from build123d import *

# Parameters (mm, degrees)
F0_R     = 1.905
F1_DEPTH = 12.7


with BuildPart() as f1:
    # F0 (on Top) → F1 (new body)
    with BuildSketch(Plane.XY):
        with BuildLine():
            ThreePointArc((114.3, 88.9), (106.860512, 106.860512), (88.9, 114.3))
            Line((88.9, 114.3), (3.175, 114.3))
            Line((3.175, 114.3), (3.175, 8.980256))
            ThreePointArc((3.175, 8.980256), (6.735192, 6.735192), (8.980256, 3.175))
            Line((8.980256, 3.175), (114.3, 3.175))
            Line((114.3, 3.175), (114.3, 88.9))
        make_face()
        with Locations((12.7, 12.7)):
            Circle(F0_R, mode=Mode.SUBTRACT)
        with Locations((38.1, 12.7)):
            Circle(F0_R, mode=Mode.SUBTRACT)
        with Locations((12.7, 38.1)):
            Circle(F0_R, mode=Mode.SUBTRACT)
        with Locations((38.1, 38.1)):
            Circle(F0_R, mode=Mode.SUBTRACT)
        with Locations((63.5, 12.7)):
            Circle(F0_R, mode=Mode.SUBTRACT)
        with Locations((88.9, 12.7)):
            Circle(F0_R, mode=Mode.SUBTRACT)
        with Locations((63.5, 38.1)):
            Circle(F0_R, mode=Mode.SUBTRACT)
        with Locations((88.9, 38.1)):
            Circle(F0_R, mode=Mode.SUBTRACT)
        with Locations((12.7, 63.5)):
            Circle(F0_R, mode=Mode.SUBTRACT)
        with Locations((38.1, 63.5)):
            Circle(F0_R, mode=Mode.SUBTRACT)
        with Locations((12.7, 88.9)):
            Circle(F0_R, mode=Mode.SUBTRACT)
        with Locations((38.1, 88.9)):
            Circle(F0_R, mode=Mode.SUBTRACT)
        with Locations((63.5, 63.5)):
            Circle(F0_R, mode=Mode.SUBTRACT)
        with Locations((88.9, 63.5)):
            Circle(F0_R, mode=Mode.SUBTRACT)
        with Locations((63.5, 88.9)):
            Circle(F0_R, mode=Mode.SUBTRACT)
        with Locations((88.9, 88.9)):
            Circle(F0_R, mode=Mode.SUBTRACT)
        with BuildLine():
            Line((3.175, 8.980256), (3.175, 114.3))
            Line((3.175, 114.3), (-3.175, 114.3))
            Line((-3.175, 114.3), (-3.175, 8.980256))
            ThreePointArc((-3.175, 8.980256), (0, 9.525), (3.175, 8.980256))
        make_face()
        with BuildLine():
            Line((-3.175, 8.980256), (-3.175, 114.3))
            Line((-3.175, 114.3), (-88.9, 114.3))
            ThreePointArc((-88.9, 114.3), (-106.860512, 106.860512), (-114.3, 88.9))
            Line((-114.3, 88.9), (-114.3, 3.175))
            Line((-114.3, 3.175), (-8.980256, 3.175))
            ThreePointArc((-8.980256, 3.175), (-6.735192, 6.735192), (-3.175, 8.980256))
        make_face()
        with Locations((-88.9, 12.7)):
            Circle(F0_R, mode=Mode.SUBTRACT)
        with Locations((-63.5, 12.7)):
            Circle(F0_R, mode=Mode.SUBTRACT)
        with Locations((-88.9, 38.1)):
            Circle(F0_R, mode=Mode.SUBTRACT)
        with Locations((-63.5, 38.1)):
            Circle(F0_R, mode=Mode.SUBTRACT)
        with Locations((-38.1, 12.7)):
            Circle(F0_R, mode=Mode.SUBTRACT)
        with Locations((-12.7, 12.7)):
            Circle(F0_R, mode=Mode.SUBTRACT)
        with Locations((-38.1, 38.1)):
            Circle(F0_R, mode=Mode.SUBTRACT)
        with Locations((-12.7, 38.1)):
            Circle(F0_R, mode=Mode.SUBTRACT)
        with Locations((-88.9, 63.5)):
            Circle(F0_R, mode=Mode.SUBTRACT)
        with Locations((-63.5, 63.5)):
            Circle(F0_R, mode=Mode.SUBTRACT)
        with Locations((-88.9, 88.9)):
            Circle(F0_R, mode=Mode.SUBTRACT)
        with Locations((-63.5, 88.9)):
            Circle(F0_R, mode=Mode.SUBTRACT)
        with Locations((-38.1, 63.5)):
            Circle(F0_R, mode=Mode.SUBTRACT)
        with Locations((-12.7, 63.5)):
            Circle(F0_R, mode=Mode.SUBTRACT)
        with Locations((-38.1, 88.9)):
            Circle(F0_R, mode=Mode.SUBTRACT)
        with Locations((-12.7, 88.9)):
            Circle(F0_R, mode=Mode.SUBTRACT)
        with BuildLine():
            Line((114.3, -3.175), (114.3, 3.175))
            Line((114.3, 3.175), (8.980256, 3.175))
            ThreePointArc((8.980256, 3.175), (9.387826, 1.610696), (9.525, 0))
            ThreePointArc((9.525, 0), (9.387826, -1.610696), (8.980256, -3.175))
            Line((8.980256, -3.175), (114.3, -3.175))
        make_face()
        with BuildLine():
            Line((114.3, -88.9), (114.3, -3.175))
            Line((114.3, -3.175), (8.980256, -3.175))
            ThreePointArc((8.980256, -3.175), (6.735192, -6.735192), (3.175, -8.980256))
            Line((3.175, -8.980256), (3.175, -114.3))
            Line((3.175, -114.3), (88.9, -114.3))
            ThreePointArc((88.9, -114.3), (106.860512, -106.860512), (114.3, -88.9))
        make_face()
        with Locations((12.7, -88.9)):
            Circle(F0_R, mode=Mode.SUBTRACT)
        with Locations((38.1, -88.9)):
            Circle(F0_R, mode=Mode.SUBTRACT)
        with Locations((12.7, -63.5)):
            Circle(F0_R, mode=Mode.SUBTRACT)
        with Locations((38.1, -63.5)):
            Circle(F0_R, mode=Mode.SUBTRACT)
        with Locations((63.5, -88.9)):
            Circle(F0_R, mode=Mode.SUBTRACT)
        with Locations((88.9, -88.9)):
            Circle(F0_R, mode=Mode.SUBTRACT)
        with Locations((63.5, -63.5)):
            Circle(F0_R, mode=Mode.SUBTRACT)
        with Locations((88.9, -63.5)):
            Circle(F0_R, mode=Mode.SUBTRACT)
        with Locations((12.7, -38.1)):
            Circle(F0_R, mode=Mode.SUBTRACT)
        with Locations((38.1, -38.1)):
            Circle(F0_R, mode=Mode.SUBTRACT)
        with Locations((12.7, -12.7)):
            Circle(F0_R, mode=Mode.SUBTRACT)
        with Locations((38.1, -12.7)):
            Circle(F0_R, mode=Mode.SUBTRACT)
        with Locations((63.5, -38.1)):
            Circle(F0_R, mode=Mode.SUBTRACT)
        with Locations((88.9, -38.1)):
            Circle(F0_R, mode=Mode.SUBTRACT)
        with Locations((63.5, -12.7)):
            Circle(F0_R, mode=Mode.SUBTRACT)
        with Locations((88.9, -12.7)):
            Circle(F0_R, mode=Mode.SUBTRACT)
        with BuildLine():
            ThreePointArc((-8.980256, -3.175), (-9.525, 0), (-8.980256, 3.175))
            Line((-8.980256, 3.175), (-114.3, 3.175))
            Line((-114.3, 3.175), (-114.3, -3.175))
            Line((-114.3, -3.175), (-8.980256, -3.175))
        make_face()
        with BuildLine():
            ThreePointArc((-3.175, -8.980256), (-6.735192, -6.735192), (-8.980256, -3.175))
            Line((-8.980256, -3.175), (-114.3, -3.175))
            Line((-114.3, -3.175), (-114.3, -88.9))
            ThreePointArc((-114.3, -88.9), (-106.860512, -106.860512), (-88.9, -114.3))
            Line((-88.9, -114.3), (-3.175, -114.3))
            Line((-3.175, -114.3), (-3.175, -8.980256))
        make_face()
        with Locations((-88.9, -88.9)):
            Circle(F0_R, mode=Mode.SUBTRACT)
        with Locations((-63.5, -88.9)):
            Circle(F0_R, mode=Mode.SUBTRACT)
        with Locations((-88.9, -63.5)):
            Circle(F0_R, mode=Mode.SUBTRACT)
        with Locations((-63.5, -63.5)):
            Circle(F0_R, mode=Mode.SUBTRACT)
        with Locations((-38.1, -88.9)):
            Circle(F0_R, mode=Mode.SUBTRACT)
        with Locations((-12.7, -88.9)):
            Circle(F0_R, mode=Mode.SUBTRACT)
        with Locations((-38.1, -63.5)):
            Circle(F0_R, mode=Mode.SUBTRACT)
        with Locations((-12.7, -63.5)):
            Circle(F0_R, mode=Mode.SUBTRACT)
        with Locations((-88.9, -38.1)):
            Circle(F0_R, mode=Mode.SUBTRACT)
        with Locations((-63.5, -38.1)):
            Circle(F0_R, mode=Mode.SUBTRACT)
        with Locations((-88.9, -12.7)):
            Circle(F0_R, mode=Mode.SUBTRACT)
        with Locations((-63.5, -12.7)):
            Circle(F0_R, mode=Mode.SUBTRACT)
        with Locations((-38.1, -38.1)):
            Circle(F0_R, mode=Mode.SUBTRACT)
        with Locations((-12.7, -38.1)):
            Circle(F0_R, mode=Mode.SUBTRACT)
        with Locations((-38.1, -12.7)):
            Circle(F0_R, mode=Mode.SUBTRACT)
        with Locations((-12.7, -12.7)):
            Circle(F0_R, mode=Mode.SUBTRACT)
        with BuildLine():
            Line((3.175, -114.3), (3.175, -8.980256))
            ThreePointArc((3.175, -8.980256), (0, -9.525), (-3.175, -8.980256))
            Line((-3.175, -8.980256), (-3.175, -114.3))
            Line((-3.175, -114.3), (3.175, -114.3))
        make_face()
    extrude(amount=-F1_DEPTH)


solid = f1.part
Can you work these out from the model? Positions are in its coordinate system, mm. Give positions to 0.01 mm unless a question says otherwise; leave off trailing zeros. Answer as a JSON object with one key per item and string values. Group by question number.
Item 1: Suppose I cut it at A-A (z = -3.75). State how many separate pieces and enclosed holes the cut face has, plus the area to 3 significant figures.
Item 2: I'm going to push a flat-ended pin straight in: P1, Ø6, axis at x = 38.1, y = 12.7, coming from the -Z side. Where does the tip first touch, or does it pass through?
Item 3: Please list where this line runs through material, in increasing order: line 1 (X direction, y = -6.5, z = -5.5). Write a range as [from, to].
Findings:
{
 "1": {"separate pieces": "1", "enclosed holes": "65", "area": "50,700 mm²"},
 "2": {"P1": "stops at z = -12.7"},
 "3": {"line 1": "x = [-114.3, -6.96], [6.96, 114.3]"}
}
